Check sheet for the modelled part. Datum: model origin and axes. Units: mm. Face numbers are marked on the shaded views. Give positions to 0.01 mm unless a question says otherwise; leave off trailing zeros. Loops run counter-clockwise (first coordinate to the right, second up) from the corner with the lowest first, then second, coordinate; pieces in that order, holes last. Notation, with made-up numbers: M 75.25,53 L 88.25,53 A10 cw 88.25,63 Z; hole C 67,28 d4. An arc over 180 degrees is marked long. One line per question, with ' | ' between items. Start each with the question number.
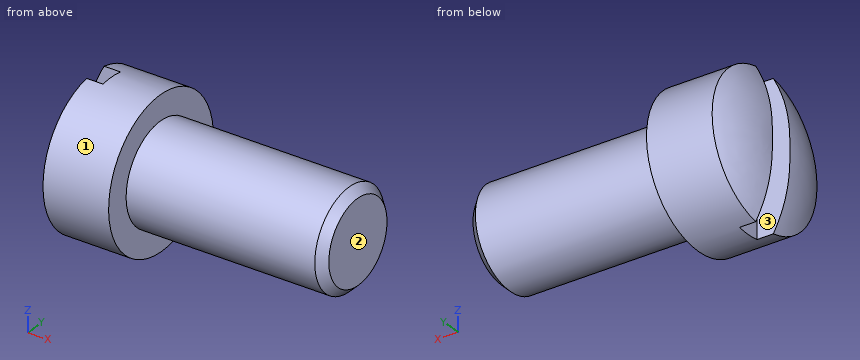
from build123d import *

# Parameters (mm, degrees)
CUT_EXTRUDE1_DEPTH      = 22.567344827
CUT_EXTRUDE1_DEPTH_BACK = 22.567344827
SKETCH2_W               = 3.175
SKETCH2_H               = 2.3876
CHAMFER1_SIZE           = 0.79375


with BuildPart() as part:
    # Sketch1 → Revolve1 (revolve)
    with BuildSketch(Plane.XY, mode=Mode.PRIVATE) as revolve1_sk:
        with BuildLine():
            Line((-4.7752, 0), (19.05, 0))
            Line((19.05, 0), (19.05, 4.7625))
            Line((19.05, 4.7625), (0, 4.7625))
            Line((0, 4.7625), (0, 7.1501))
            Line((0, 7.1501), (-6.35, 7.1501))
            ThreePointArc((-6.35, 7.1501), (-7.543180771, 4.277553789), (-7.9502, 1.1938))
            Line((-7.9502, 1.1938), (-4.7752, 1.1938))
            Line((-4.7752, 1.1938), (-4.7752, 0))
        make_face()
    revolve(revolve1_sk.sketch.rotate(Axis((25.63827619, 0, 0), (-1, 0, 0)), 90), axis=Axis((25.63827619, 0, 0), (-1, 0, 0)))

    # Sketch2 → Cut-Extrude1 (cut, two sides: drawn at the far end of the back side and taken through both)
    with BuildSketch(Plane.XY.offset(-CUT_EXTRUDE1_DEPTH_BACK)):
        with Locations((-6.3627, 0)):
            Rectangle(SKETCH2_W, SKETCH2_H)
    extrude(amount=CUT_EXTRUDE1_DEPTH + CUT_EXTRUDE1_DEPTH_BACK, mode=Mode.SUBTRACT)

    # Chamfer1
    chamfer1_edges = [part.edges().sort_by_distance(p)[0] for p in [
        (19.05, 0, 4.7625),
    ]]
    chamfer(chamfer1_edges, length=CHAMFER1_SIZE)


solid = part.part
Q1. Material ranges on probe 1 along X at (y, z) = (-1, -0.5); probe 2 along Y at (x, z) = (-6, 4.25); probe 3 along Y at (x, z) = (-5, 3), recorded low to high. Write a range as from..to.
Q2. Draft check along Y on the marked faces 1, 2 and 3. Enter one of: released by +Y, released by -Y, zero draft, split by the parting line, or undercut.
Q3. Cross-section at C-C (x = 9.5). Record the cut outline in (y, z) (1 decimal), and give its area (3 significant figures).
Q4. Depth check by flat-ended pin: P1, Ø2, axis at y = 1, z = 2, coming from the -X side; P2, Ø6, axis at y = -5.5, z = 2, coming from the +X side; P3, Ø1.5, axis at x = 8.5, z = -4.5, coming from the -Y side; P4, Ø2, axis at x = 11, z = -2, coming from the -Y side. Enter the tip coordinate at first touch or a pass-through.
Q5. Cross-section at A-A (y = 0). Record the cut outline in (x, z).
Q6. Cross-section at B-B (x = -2.5). Record the cut outline in (y, z).
Solved:
1) probe 1: x = -4.78..19.05 | probe 2: y = -5.75..-1.19, 1.19..5.75 | probe 3: y = -6.49..-1.19, 1.19..6.49
2) face 1: split by the parting line | face 2: zero draft | face 3: undercut
3) outline: C 0,0 d9.5 | area: 71.3 mm²
4) P1: stops at x = -7.94 | P2: stops at x = 19.05 | P3: stops at y = -2.94 | P4: stops at y = -4.66
5) outline: M -4.78,-7.15 L 0,-7.15 L 0,-4.76 L 18.26,-4.76 L 19.05,-3.97 L 19.05,3.97 L 18.26,4.76 L 0,4.76 L 0,7.15 L -4.78,7.15 Z
6) outline: C 0,0 d14.3
